from build123d import *

# Parameters (mm, degrees)
SKETCH_1_W           = 2.7
SKETCH_1_H           = 3.5
EXTRUDE_1_DEPTH      = 3.8
SKETCH_2_OUTSIDE_W   = 5.866
SKETCH_2_OUTSIDE_H   = 6.666
SKETCH_2_OUTSIDE_W_2 = 2.7
SKETCH_2_OUTSIDE_H_2 = 3.5
SKETCH_2_OUTSIDE_R   = 1
CUT_EXTRUDE_1_DEPTH  = 5.396020928
SKETCH_4_OUTSIDE_W   = 5.866
SKETCH_4_OUTSIDE_H   = 6.966
SKETCH_4_OUTSIDE_W_2 = 2.7
SKETCH_4_OUTSIDE_H_2 = 3.8
SKETCH_4_OUTSIDE_R   = 0.75
CUT_EXTRUDE_2_DEPTH  = 1.85
SKETCH_7_R           = 1.2
EXTRUDE_3_DEPTH      = 1
SKETCH_8_R           = 0.4
EXTRUDE_4_DEPTH      = 3.75
FILLET_1_R           = 0.1
FILLET_2_R           = 0.1
FILLET_3_R           = 0.1
FILLET_4_R           = 0.2


with BuildPart() as part:
    # Эскиз1 → Бобышка-Вытянуть1 (new body)
    with BuildSketch(Plane.XY):
        Rectangle(SKETCH_1_W, SKETCH_1_H)
    extrude(amount=-EXTRUDE_1_DEPTH)

    # Эскиз2 outside → Вырез-Вытянуть1 (cut, through all)
    # profile 1 of 2: a face of its own
    with BuildSketch(Plane.XY):
        Rectangle(SKETCH_2_OUTSIDE_W, SKETCH_2_OUTSIDE_H)
        Rectangle(SKETCH_2_OUTSIDE_W_2, SKETCH_2_OUTSIDE_H_2, mode=Mode.SUBTRACT)
    # profile 2 of 2: a face of its own
    with BuildSketch(Plane.XY):
        with Locations((0, -0.3)):
            Circle(SKETCH_2_OUTSIDE_R)
    extrude(amount=-CUT_EXTRUDE_1_DEPTH, mode=Mode.SUBTRACT)

    # Эскиз4 outside → Вырез-Вытянуть2 (cut)
    # profile 1 of 2: a face of its own
    with BuildSketch(Plane(origin=(0, 1.75, 0), x_dir=(1, 0, 0), z_dir=(0, 1, 0))):
        with Locations((0, 1.9)):
            Rectangle(SKETCH_4_OUTSIDE_W, SKETCH_4_OUTSIDE_H)
        with Locations((0, 1.9)):
            Rectangle(SKETCH_4_OUTSIDE_W_2, SKETCH_4_OUTSIDE_H_2, mode=Mode.SUBTRACT)
    # profile 2 of 2: a face of its own
    with BuildSketch(Plane(origin=(0, 1.75, 0), x_dir=(1, 0, 0), z_dir=(0, 1, 0))):
        with Locations(Location((0, 2, 0), (0, 0, 270))):
            Circle(SKETCH_4_OUTSIDE_R)
    extrude(amount=-CUT_EXTRUDE_2_DEPTH, mode=Mode.SUBTRACT)

    # Эскиз7 → Бобышка-Вытянуть3 (add)
    with BuildSketch(Plane.XY):
        with Locations((0, -0.3)):
            Circle(SKETCH_7_R)
    extrude(amount=EXTRUDE_3_DEPTH)

    # Эскиз8 → Бобышка-Вытянуть4 (add)
    with BuildSketch(Plane.XY.offset(1)):
        with Locations((0, -0.3)):
            Circle(SKETCH_8_R)
    extrude(amount=EXTRUDE_4_DEPTH)

    # Скругление1
    fillet_1_edges = [part.edges().sort_by_distance(p)[0] for p in [
        (-1.2, -0.3, 1),
    ]]
    fillet(fillet_1_edges, radius=FILLET_1_R)

    # Скругление2
    fillet_2_edges = [part.edges().sort_by_distance(p)[0] for p in [
        (-1.2, -0.3, 0),
    ]]
    fillet(fillet_2_edges, radius=FILLET_2_R)

    # Скругление3
    fillet_3_edges = [part.edges().sort_by_distance(p)[0] for p in [
        (-0.4, -0.3, 1),
    ]]
    fillet(fillet_3_edges, radius=FILLET_3_R)

    # Скругление4
    fillet_4_edges = [part.edges().sort_by_distance(p)[0] for p in [
        (-0.4, -0.3, 4.75),
    ]]
    fillet(fillet_4_edges, radius=FILLET_4_R)


solid = part.part
Read the model definition and answer for the solid it produces. Units are mm, in the model's axes. A direction names the side the tool comes from. Round coordinates to 2 decimals unless told otherwise and drop trailing zeros. Order: outer loops, then holes, each group sorted by start corner. A loop starts at its lowest first (then second) coordinate and runs counter-clockwise, first axis right, second up.
1) The part is cut by section A-A on z = -0.5. Write down the section's boundary in (x, y).
2) Flat-ended cylindrical pins translate along their axes: pin 1 (1 mm diameter, centred on x = -1, y = -0.5, fed in from +Z); pin 2 (1 mm diameter, centred on x = 0, y = 0, fed in from -Z). Find the tip coordinate at first contact, or state that the pin passes through.
3) The mould has two halves that part along Z. Classify faces 4 (the face through (-1.35, 0, -2)), 5 (the face through (-0.456, 1.065, -2.595)), 6 (the face through (0, 0, 0)), 7 (the face through (0, -1, 1)): released by +Z, released by -Z, zero draft, split by the parting line, or undercut.
4) Straight lines are drawn through the part: L1, parallel to Z at x = 0, y = 0.75; L2, parallel to X at y = 1.2, z = -2; L3, parallel to X at y = -0.3, z = -1.1. For each, find the intervals that lie inside material, in ascending order.
5) The part is cut by section D-D on z = 3.75. Write down the section's boundary in (x, y), plus the area to 3 significant figures.
6) The part is cut by section C-C on z = -2. Write down the section's boundary in (x, y), plus the area to 3 significant figures.
7) For faces 1 (the face through (-0.217, -1.276, -1.873)), 2 (the face through (1.35, 0, -2)), 3 (the face through (0.65, 0.71, 0.49)), determine the directions among +Z, -Z, +X, -X, +Y, -Y from which every point of the face is accessible in a straight line to the end or side of a thin tool.
8) The part is cut by section B-B on y = 1.15. Write down the section's boundary in (x, z), plus the area to 3 significant figures.
Resolved:
1. outline: (-1.35, -1.75) - (1.35, -1.75) - (1.35, 1.75) - (-1.35, 1.75) - close; hole circle Ø2 at (0, -0.3)
2. pin 1: stops at z = 1
2. pin 2: stops at z = 0
3. face 4: zero draft
3. face 5: undercut
3. face 6: released by -Z
3. face 7: released by +Z
4. L1: z = -3.8 to -2.75, -1.25 to 1
4. L2: x = -1.35 to -0.75, 0.75 to 1.35
4. L3: x = -1.35 to -1, 1 to 1.35
5. outline: circle Ø0.8 at (0, -0.3)
5. area: 0.503 mm2
6. outline: (-1.35, -1.75) - (1.35, -1.75) - (1.35, 1.75) - (0.75, 1.75) - (0.75, 0.36) arc R1 cw (long way) to (-0.75, 0.36) - (-0.75, 1.75) - (-1.35, 1.75) - close
6. area: 4.58 mm2
7. face 1: -Z
7. face 2: +Z, -Z, +X, +Y, -Y
7. face 3: +Z
8. outline: (-1.35, -3.8) - (1.35, -3.8) - (1.35, 0) - (-1.35, 0) - close; hole circle Ø1.5 at (0, -2)
8. area: 8.49 mm2
